Source: three-view drawing plus pictorial views. Frame: mm from the lowest corner of the part. A direction names the side the tool comes from. Give positions to 0.01 mm unless a question says otherwise; leave off trailing zeros. Order: outer loops, then holes, each group sorted by start corner. A loop starts at its lowest first (then second) coordinate and runs counter-clockwise, first axis right, second up. Notation, with made-up numbers: M -36.75,23 L 11.25,23 A29 ccw 11.25,52 Z; hole C 23.5,-39.5 d10. An arc over 180 degrees is marked long. One line per item, written item: value. Start each with the question number.
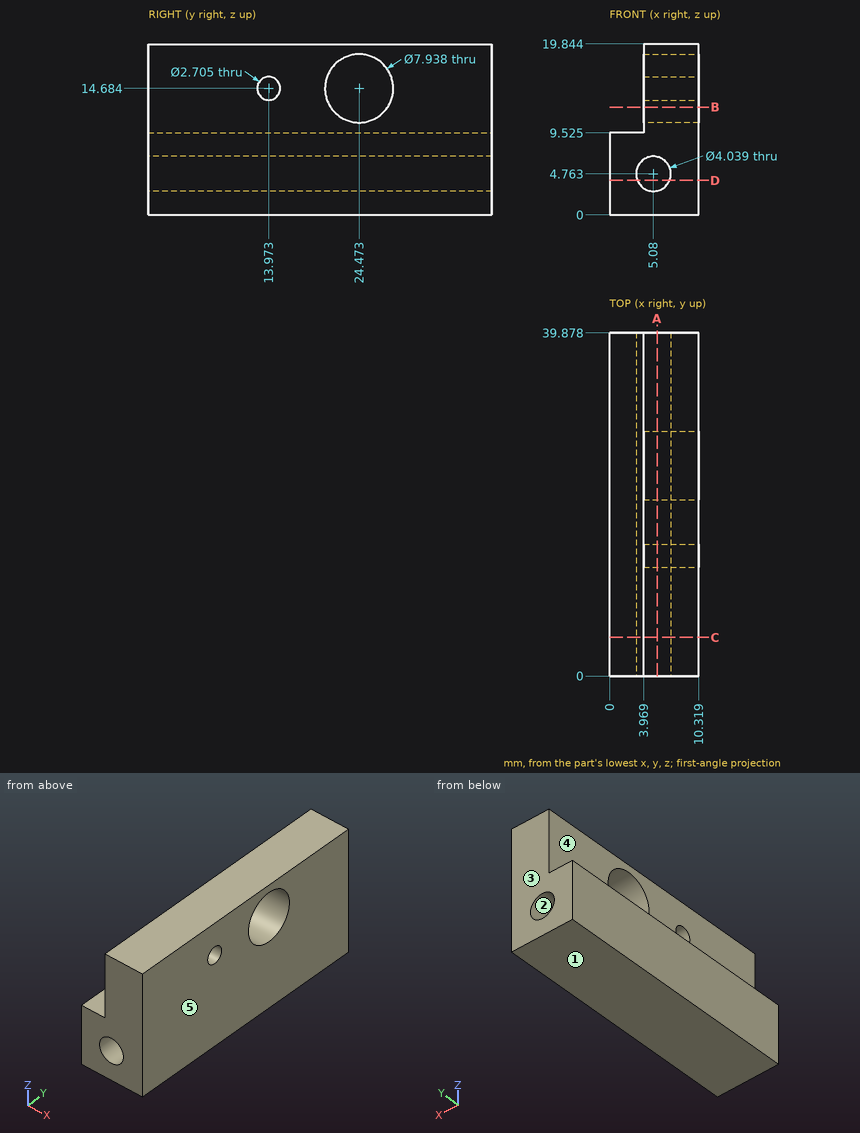
Q1. Mould query, pull axis Z, two halves, no side actions, for the marked faces 1, 2 and 3. Classes: +Z half, -Z half, draft (parallel to the pull), parting line (faces both ways), or undercut.
Q2. Set-up query: the marked faces 4 and 5. Return all of +Z, -Z, +X, -X, +Y, -Y with unobstructed straight access to the full face (end or side cutting, diameter ignored); none if empty.
Q3. Contact query for flat-ended pins moving along their axis: pin 1 (3 mm diameter, centred on y = 13.97, z = 14.68, fed in from -X); pin 2 (1.2 mm diameter, centred on x = 2.5, y = 12.5, fed in from +Z) (1 decimal). Output: stop coordinate, or through.
Q4. Section query C-C on y = 4.5. Return loops of the section in (x, z) (1 decimal).
Q5. Section query D-D on z = 4. Return loops of the section in (x, y).
Q6. Section query B-B on z = 12.5. Return loops of the section in (x, y).
Q7. Ray query, line 1 along Z through (x, y) = (6, 14.5) (1 decimal); line 2 along Z through (x, y) = (1, 3.5) (1 decimal); line 3 along X through (y, z) = (34.5, 16.5). Return the intervals inside material, ascending. Write a range as [from, to].
Q8. Section query A-A on x = 5.5. Return loops of the section in (y, z) (1 decimal).
Results below:
1. face 1: -Z half
1. face 2: undercut
1. face 3: draft
2. face 4: +Z, -X, +Y, -Y
2. face 5: +Z, -Z, +X, +Y, -Y
3. pin 1: x = 3.97
3. pin 2: z = 9.5
4. outline: M 0,0 L 10.3,0 L 10.3,19.8 L 4,19.8 L 4,9.5 L 0,9.5 Z; hole C 5.1,4.8 d4
5. outline: M 0,0 L 3.21,0 L 3.21,39.88 L 0,39.88 Z; M 6.95,0 L 10.32,0 L 10.32,39.88 L 6.95,39.88 Z
6. outline: M 3.97,0 L 10.32,0 L 10.32,21.16 L 3.97,21.16 Z; M 3.97,27.79 L 10.32,27.79 L 10.32,39.88 L 3.97,39.88 Z
7. line 1: [0, 3], [6.6, 13.4], [15.9, 19.8]
7. line 2: [0, 9.5]
7. line 3: [3.97, 10.32]
8. outline: M 0,0 L 39.9,0 L 39.9,2.8 L 0,2.8 Z; M 0,6.7 L 39.9,6.7 L 39.9,19.8 L 0,19.8 Z; hole C 14,14.7 d2.7; hole C 24.5,14.7 d7.9
